Could you check a few things on this model? Use its own coordinates, in mm. Face numbers are marked on the shaded views. A direction names the side the tool comes from. Round coordinates to 2 decimals unless told otherwise and drop trailing zeros. Loops run counter-clockwise (first coordinate to the right, second up) from the corner with the lowest first, then second, coordinate; pieces in that order, holes last.
from build123d import *

# Parameters (mm, degrees)
SKETCH6_W                = 230
SKETCH6_H                = 30
BOSS_EXTRUDE1_DEPTH      = 9.5
BOSS_EXTRUDE2_DEPTH      = 9.5
BOSS_EXTRUDE2_DEPTH_BACK = 25
SKETCH12_R               = 6.5
CUT_EXTRUDE2_DEPTH       = 2
SKETCH15_R               = 6.5
CUT_EXTRUDE3_DEPTH       = 2
CUT_EXTRUDE4_DEPTH       = 6
SKETCH9_W                = 4.5
SKETCH9_H                = 12
CUT_EXTRUDE5_DEPTH       = 231
SKETCH17_W               = 5
SKETCH17_H               = 12
CUT_EXTRUDE6_DEPTH       = 29.5
SKETCH13_R               = 1.75
CUT_EXTRUDE8_DEPTH       = 16
SKETCH19_W               = 3
SKETCH19_H               = 5.6
CUT_EXTRUDE9_DEPTH       = 10
SKETCH20_W               = 4
SKETCH20_H               = 4
BOSS_EXTRUDE3_DEPTH      = 9.5
SKETCH20_3_W             = 25
SKETCH20_3_H             = 4
SKETCH20_3_W_2           = 4
CUT_EXTRUDE10_DEPTH      = 9.3
CUT_EXTRUDE11_DEPTH      = 10.5
CHAMFER2_SIZE            = 2.1
CHAMFER3_SIZE            = 2


with BuildPart() as part:
    # Sketch6 → Boss-Extrude1 (new body)
    with BuildSketch(Plane.XY):
        with Locations((-184.090144231, 89)):
            Rectangle(SKETCH6_W, SKETCH6_H)
    extrude(amount=BOSS_EXTRUDE1_DEPTH)

    # Sketch11 → Boss-Extrude2 (add, two sides)
    with BuildSketch(Plane.XY) as boss_extrude2_sk:
        Polygon((-299.090144231, 74), (-288.092548077, 104), (-314.090144231, 104), (-314.090144231, 74), align=None)
    extrude(amount=BOSS_EXTRUDE2_DEPTH)
    extrude(boss_extrude2_sk.sketch, amount=-BOSS_EXTRUDE2_DEPTH_BACK)

    # Sketch12 → Cut-Extrude2 (cut)
    with BuildSketch(Plane.ZY.offset(314.090144231)):
        with Locations((1.5, 89)):
            Circle(SKETCH12_R)
    extrude(amount=-CUT_EXTRUDE2_DEPTH, mode=Mode.SUBTRACT)

    # Sketch15 → Cut-Extrude3 (cut)
    with BuildSketch(Plane(origin=(0, 0, 0), x_dir=(-1, 0, 0), z_dir=(0, 0, -1))):
        with Locations((158.090144231, 89)):
            Circle(SKETCH15_R)
    extrude(amount=-CUT_EXTRUDE3_DEPTH, mode=Mode.SUBTRACT)

    # Sketch16 → Cut-Extrude4 (cut)
    with BuildSketch(Plane(origin=(0, 0, -25), x_dir=(-1, 0, 0), z_dir=(0, 0, -1))):
        Polygon((303.890144231, 74), (303.890144231, 104), (288.092548077, 104), (299.090144231, 74), align=None)
    extrude(amount=-CUT_EXTRUDE4_DEPTH, mode=Mode.SUBTRACT)

    # Sketch9 → Cut-Extrude5 (cut, through all)
    with BuildSketch(Plane.ZY.offset(299.090144231)):
        with Locations((5.25, 89)):
            Rectangle(SKETCH9_W, SKETCH9_H)
    extrude(amount=-CUT_EXTRUDE5_DEPTH, mode=Mode.SUBTRACT)

    # Sketch17 → Cut-Extrude6 (cut, through all)
    with BuildSketch(Plane(origin=(0, 0, -19), x_dir=(-1, 0, 0), z_dir=(0, 0, -1))):
        with Locations((301.390144231, 89)):
            Rectangle(SKETCH17_W, SKETCH17_H)
    extrude(amount=-CUT_EXTRUDE6_DEPTH, mode=Mode.SUBTRACT)

    # Sketch13 → Cut-Extrude8 (cut)
    with BuildSketch(Plane(origin=(0, 0, -25), x_dir=(-1, 0, 0), z_dir=(0, 0, -1))):
        with Locations((307.640144231, 79)):
            Circle(SKETCH13_R)
        with Locations((307.640144231, 99)):
            Circle(SKETCH13_R)
    extrude(amount=-CUT_EXTRUDE8_DEPTH, mode=Mode.SUBTRACT)

    # Sketch19 → Cut-Extrude9 (cut)
    with BuildSketch(Plane.ZY.offset(314.090144231)):
        with Locations((-14.5, 79)):
            Rectangle(SKETCH19_W, SKETCH19_H)
        with Locations((-14.5, 99)):
            Rectangle(SKETCH19_W, SKETCH19_H)
    extrude(amount=-CUT_EXTRUDE9_DEPTH, mode=Mode.SUBTRACT)

    # Sketch20 → Boss-Extrude3 (add)
    with BuildSketch(Plane(origin=(0, 0, 0), x_dir=(-1, 0, 0), z_dir=(0, 0, -1))):
        Polygon((69.090144231, 101), (69.090144231, 104), (69.090144231, 107), (65.090144231, 104), (65.090144231, 101), align=None)
        with Locations((67.090144231, 99)):
            Rectangle(SKETCH20_W, SKETCH20_H)
    extrude(amount=-BOSS_EXTRUDE3_DEPTH)

    # Sketch20<3> → Cut-Extrude10 (cut)
    with BuildSketch(Plane(origin=(0, 0, 0), x_dir=(-1, 0, 0), z_dir=(0, 0, -1))):
        with Locations((81.590144231, 99)):
            Rectangle(SKETCH20_3_W, SKETCH20_3_H)
        with Locations((67.090144231, 99)):
            Rectangle(SKETCH20_3_W_2, SKETCH20_3_H)
    extrude(amount=-CUT_EXTRUDE10_DEPTH, mode=Mode.SUBTRACT)

    # Sketch21 → Cut-Extrude11 (cut, through all)
    with BuildSketch(Plane(origin=(0, 0, 0), x_dir=(-1, 0, 0), z_dir=(0, 0, -1))):
        Polygon((288.092548077, 104), (288.184194712, 103.75), (69.090144231, 103.75), (69.090144231, 104), align=None)
        Polygon((299.090144231, 74), (69.090144231, 74), (69.090144231, 74.25), (298.998497596, 74.25), align=None)
    extrude(amount=-CUT_EXTRUDE11_DEPTH, mode=Mode.SUBTRACT)

    # Chamfer2
    chamfer2_edges = [part.edges().sort_by_distance(p)[0] for p in [
        (-178.637169471, 103.75, 9.5),
        (-178.637169471, 103.75, 0),
        (-184.044320913, 74.25, 9.5),
        (-184.044320913, 74.25, 0),
    ]]
    chamfer(chamfer2_edges, length=CHAMFER2_SIZE)

    # Chamfer3
    chamfer3_edges = [part.edges().sort_by_distance(p)[0] for p in [
        (-301.091346154, 104, 9.5),
        (-306.590144231, 74, 9.5),
    ]]
    chamfer(chamfer3_edges, length=CHAMFER3_SIZE)


solid = part.part
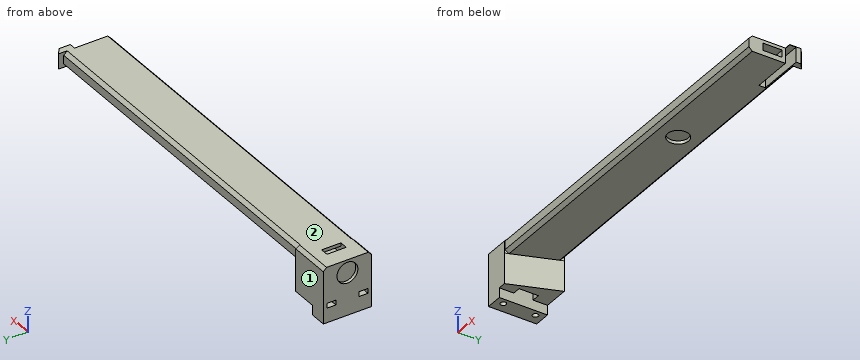
Item 1: If I drill on line 1 along Z through (x, y) = (-157, 89.5); line 2 along Z through (x, y) = (-254.5, 84); line 3 along X through (y, z) = (94, 1.5), over which ranges is the centre line in solid material (lowest first)?
Results list:
line 1: z = 2 to 3, 7.5 to 9.5
line 2: z = 0 to 3, 7.5 to 9.5
line 3: x = -312.09 to -303.89, -298.89 to -162.24, -153.94 to -69.09
Item 2: If we section it at C-C, the plane y = 89: Please give me the cut outline in (x, z), then the cut area to 3 significant figures.
Results list:
outline: (-314.09, -25) - (-303.89, -25) - (-303.89, 9.5) - (-314.09, 9.5) - (-314.09, 8) - (-312.09, 8) - (-312.09, -5) - (-314.09, -5) - close; (-298.89, -19) - (-293.59, -19) - (-293.59, 0) - (-164.59, 0) - (-164.59, 2) - (-151.59, 2) - (-151.59, 0) - (-69.09, 0) - (-69.09, 3) - (-298.89, 3) - close; (-298.89, 7.5) - (-69.09, 7.5) - (-69.09, 9.5) - (-298.89, 9.5) - close
area: 1,550 mm2
Item 3: Will these pins go through, and if not, where does the flat tip stop? pin 1 (1.5 mm diameter, centred on x = -308.5, z = -14, fed in from +Y); pin 2 (4 mm diameter, centred on x = -157.5, y = 90.5, fed in from -Z); pin 3 (12 mm diameter, centred on x = -143, y = 95.5, fed in from -Z); pin 4 (12 mm diameter, centred on x = -259.5, z = -11.5, fed in from +Y).
Results list:
pin 1: stops at y = 104
pin 2: stops at z = 2
pin 3: stops at z = 0
pin 4: passes through
Item 4: If we section it at A-A, the plane z = -21.5: Please give me the cut outline in (x, y), then the cut area to 3 significant figures.
Results list:
outline: (-314.09, 74) - (-303.89, 74) - (-303.89, 104) - (-314.09, 104) - close; hole circle Ø3.5 at (-307.64, 79); hole circle Ø3.5 at (-307.64, 99)
area: 287 mm2
Item 5: If we section it at B-B, the plane x = -176: Please give me the cut outline in (y, z).
Results list:
outline: (74.25, 2.1) - (76.35, 0) - (101.65, 0) - (103.75, 2.1) - (103.75, 7.4) - (101.65, 9.5) - (76.35, 9.5) - (74.25, 7.4) - close; hole (83, 3) - (95, 3) - (95, 7.5) - (83, 7.5) - close
Item 6: For the marked faces 1 and 2, which set-ups out of +Z, -Z, +X, -X, +Y, -Y let a thin tool reach every point of the face, with its end or its side?
Results list:
face 1: +Z, -Z, -X, +Y
face 2: +Z, +X, -X, +Y, -Y
